from build123d import *

# Parameters (mm, degrees)
F0_R     = 23.0531460168
F1_DEPTH = 82
F1_TAPER = -10
F2_T     = -3
F3_R     = 1


with BuildPart() as f1:
    # F0 (on Top) → F1 (new body)
    with BuildSketch(Plane.XY):
        Circle(F0_R)
    extrude(amount=F1_DEPTH, taper=F1_TAPER)

    # F2
    f2_openings = [f1.faces().sort_by_distance(p)[0] for p in [
        (0, 0, 82),
    ]]
    offset(amount=F2_T, openings=f2_openings, kind=Kind.INTERSECTION)

    # F3
    f3_edges = [f1.edges().sort_by_distance(p)[0] for p in [
        (-37.511958, 0, 82),
        (-34.465679, 0, 82),
        (-23.053146, 0, 0),
    ]]
    fillet(f3_edges, radius=F3_R)


solid = f1.part
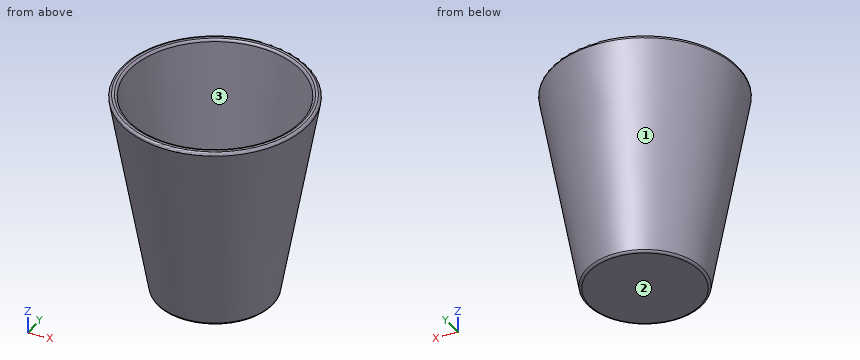
Here's how the part is built. I have some questions about the finished solid (model axes, mm). Face numbers are marked on the shaded views. Coordinates: 2 decimals unless noted, no trailing zeros. Order: outer loops, then holes, each group sorted by start corner. A loop starts at its lowest first (then second) coordinate and runs counter-clockwise, first axis right, second up. Notation, with made-up numbers: M -16.5,44 L 32.5,44 A7 ccw 32.5,51 Z; hole C -39,28.25 d6. An arc over 180 degrees is marked long. Answer as CSV lines item,"result". Start each with the question number.
1. I need wall thicknesses on line 1 (Z direction, x = 5, y = -15); line 2 (Y direction, x = -24, z = 50.5); line 3 (X direction, y = 22.5, z = 50.5). Which ranges of each line are inside material? Lowest first, please. Write a range as [from, to].
2. I want a section at C-C, the plane z = 68. Write out the boundary of the cut face in (x, y).
3. I want a section at B-B, the plane z = 17. Write out the boundary of the cut face in (x, y), and give its area (3 significant figures).
4. For pin 1 (3 mm diameter, centred on y = 19.5, z = 25, fed in from +X); pin 2 (1 mm diameter, centred on x = -23.5, z = 35.5, fed in from -Y); pin 3 (1 mm diameter, centred on x = -15, z = 67, fed in from -Y), each with a flat end and sliding along its axis, tell me the tip position at first contact or that it passes through.
5. We'd pull the mould along X, two halves only. Please class the marked faces 1, 2 and 3: released by +X, released by -X, zero draft, split by the parting line, or undercut.
6. I want a section at A-A, the plane x = 0. Write out the boundary of the cut face in (y, z), and give its area (3 significant figures).
Recorded:
1,line 1,"z = [0, 3]"
1,line 2,"y = [-21.1, -16.12], [16.12, 21.1]"
1,line 3,"x = [-22.69, -18.16], [18.16, 22.69]"
2,outline,"C 0,0 d70.09; hole C 0,0 d63.99"
3,outline,"C 0,0 d52.1; hole C 0,0 d46.01"
3,area,"469 mm2"
4,pin 1,"stops at x = 20.79"
4,pin 2,"stops at y = -18.19"
4,pin 3,"stops at y = -31.73"
5,face 1,"split by the parting line"
5,face 2,"zero draft"
5,face 3,"undercut"
6,outline,"M -37.31,80.83 L -23.2,0.83 A1 ccw -22.21,0 L 22.21,0 A1 ccw 23.2,0.83 L 37.31,80.83 A1 ccw 36.32,82 L 35.3,82 A1 ccw 34.32,81.17 L 20.54,3 L -20.54,3 L -34.32,81.17 A1 ccw -35.3,82 L -36.32,82 A1 ccw Z"
6,area,"620 mm2"
